Part model, mm, in its own coordinate system. A direction names the side the tool comes from. Give positions to 0.01 mm unless a question says otherwise; leave off trailing zeros. Order: outer loops, then holes, each group sorted by start corner. A loop starts at its lowest first (then second) coordinate and runs counter-clockwise, first axis right, second up. Notation, with made-up numbers: (60.5, -4.5) - (91.5, -4.5) arc R24 cw to (91.5, 26.5) - close; hole circle Ø4 at (57, 2). An arc over 180 degrees is marked (long way). One line per item, written item: value.
```python
from build123d import *

# Parameters (mm, degrees)
SKETCH1_W                       = 53.34
SKETCH1_H                       = 96.52
BOSS_EXTRUDE1_DEPTH             = 1.6002
CUT_EXTRUDE1_DEPTH              = 1.6002
F_32_0_116_DIAMETER_HOLE1_D     = 2.9464
F_32_0_116_DIAMETER_HOLE1_DEPTH = 25.4
F_32_0_116_DIAMETER_HOLE1_TIP   = 0.885187864
CUT_EXTRUDE2_DEPTH              = 2.54
FILLET1_R                       = 0.635


with BuildPart() as part:
    # Sketch1 → Boss-Extrude1 (new body)
    with BuildSketch(Plane(origin=(0, 0, 0), x_dir=(1, 0, 0), z_dir=(0, 1, 0))):
        with Locations((26.67, 48.26)):
            Rectangle(SKETCH1_W, SKETCH1_H)
    extrude(amount=BOSS_EXTRUDE1_DEPTH)

    # Sketch2 → Cut-Extrude1 (cut)
    with BuildSketch(Plane(origin=(0, 1.6002, 0), x_dir=(1, 0, 0), z_dir=(0, 1, 0))):
        Polygon((10.16, 0), (10.16, 3.81), (8.61695, 3.81), (8.61695, 6.19125), (10.16, 6.19125), (10.16, 10.16), (13.4239, 10.16), (13.4239, 6.19125), (14.96695, 6.19125), (14.96695, 3.81), (13.4239, 3.81), (13.4239, 0), align=None)
        Polygon((28.30195, 96.52), (28.30195, 92.71), (29.845, 92.71), (29.845, 90.32875), (28.30195, 90.32875), (28.30195, 86.36), (25.03805, 86.36), (25.03805, 90.32875), (23.495, 90.32875), (23.495, 92.71), (25.03805, 92.71), (25.03805, 96.52), align=None)
        Polygon((39.9161, 0), (43.18, 0), (43.18, 3.81), (44.72305, 3.81), (44.72305, 6.19125), (43.18, 6.19125), (43.18, 10.16), (39.9161, 10.16), (39.9161, 6.19125), (38.37305, 6.19125), (38.37305, 3.81), (39.9161, 3.81), align=None)
        Polygon((0, 49.911), (3.81, 49.911), (3.81, 51.435), (6.19125, 51.435), (6.19125, 49.911), (10.16, 49.911), (10.16, 46.609), (6.19125, 46.609), (6.19125, 45.085), (3.81, 45.085), (3.81, 46.609), (0, 46.609), align=None)
        Polygon((53.34, 46.609), (53.34, 49.911), (49.53, 49.911), (49.53, 51.435), (47.14875, 51.435), (47.14875, 49.911), (43.18, 49.911), (43.18, 46.609), (47.14875, 46.609), (47.14875, 45.085), (49.53, 45.085), (49.53, 46.609), align=None)
    extrude(amount=-CUT_EXTRUDE1_DEPTH, mode=Mode.SUBTRACT)

    # #32 (0.116) Diameter Hole1
    with Locations(Plane(origin=(0, 1.6002, 0), x_dir=(1, 0, 0), z_dir=(0, 1, 0))):
        with Locations((4.572, 6.35), (49.53, 22.86), (49.53, 71.12), (4.572, 67.31)):
            Hole(F_32_0_116_DIAMETER_HOLE1_D / 2, depth=F_32_0_116_DIAMETER_HOLE1_DEPTH)
            with Locations((0, 0, -(F_32_0_116_DIAMETER_HOLE1_DEPTH + F_32_0_116_DIAMETER_HOLE1_TIP / 2))):  # 118° drill point
                Cone(0, F_32_0_116_DIAMETER_HOLE1_D / 2, F_32_0_116_DIAMETER_HOLE1_TIP, mode=Mode.SUBTRACT)

    # Sketch7 → Cut-Extrude2 (cut)
    with BuildSketch(Plane(origin=(0, 1.6002, 0), x_dir=(1, 0, 0), z_dir=(0, 1, 0))):
        Polygon((26.67, 71.12), (22.426456564, 64.879494947), (24.548228282, 64.879494947), (24.548228282, 57.141268682), (26.67, 57.141268682), (28.791771718, 57.141268682), (28.791771718, 64.937563076), (30.997705847, 64.937563076), align=None)
    extrude(amount=-CUT_EXTRUDE2_DEPTH, mode=Mode.SUBTRACT)

    # Fillet1
    fillet1_edges = [part.edges().sort_by_distance(p)[0] for p in [
        (26.67, 0.8001, -71.12),
        (30.997705847, 0.8001, -64.937563076),
        (28.791771718, 0.8001, -64.937563076),
        (28.791771718, 0.8001, -57.141268682),
        (24.548228282, 0.8001, -57.141268682),
        (24.548228282, 0.8001, -64.879494947),
        (22.426456564, 0.8001, -64.879494947),
    ]]
    fillet(fillet1_edges, radius=FILLET1_R)


solid = part.part
```
1) Which spindle directions (+Z, -Z, +X, -X, +Y, -Y) get a long thin tool onto all of the face, cutting with end or side? Do faces 1 (the flat face through (24.65, 0.81, -68.15)), 2 (the flat face through (26, 1.6, -49)). Say none if no direction does.
Outcome:
face 1: +Y, -Y
face 2: +Z, -Z, +X, -X, +Y
2) Cut at D-D, the plane x = 11.5. Give the cut face in (y, z), then the cut area to 3 significant figures.
Outcome:
outline: (0, -96.52) - (1.6, -96.52) - (1.6, -10.16) - (0, -10.16) - close
area: 138 mm^2
3) Cut at A-A, the plane z = -22.86. Give the cut face in (x, y).
Outcome:
outline: (0, 0) - (48.06, 0) - (48.06, 1.6) - (0, 1.6) - close; (51, 0) - (53.34, 0) - (53.34, 1.6) - (51, 1.6) - close
4) Mould opens along X. For faces 3 (the flat face through (28.77, 0.81, -68.12)), 4 (the flat face through (26, 0, -49)) say: released by +X, released by -X, zero draft, split by the parting line, or undercut.
Outcome:
face 3: undercut
face 4: zero draft
5) Cut at B-B, the plane z = -67.31. Give the cut face in (x, y).
Outcome:
outline: (0, 0) - (3.1, 0) - (3.1, 1.6) - (0, 1.6) - close; (6.05, 0) - (24.08, 0) - (24.08, 1.6) - (6.05, 1.6) - close; (29.34, 0) - (53.34, 0) - (53.34, 1.6) - (29.34, 1.6) - close
6) Pin check, flat tip, straight feed: pin 1 (0.5 mm diameter, centred on y = 0.5, z = -2, fed in from -X). Stop position of the tip, or through.
Outcome:
pin 1: stops at x = 0
7) Cut at C-C, the plane y = 0.25. Give the number of separate pieces and of enclosed holes in the cut face, then the cut area to 3 significant figures.
Outcome:
separate pieces: 1
enclosed holes: 5
area: 4,860 mm^2
8) Drill centre lines: line 1 along X through (y, z) = (0.3, -46.5); line 2 along X through (y, z) = (0.65, -89.5); line 3 along X through (y, z) = (0.7, -6.35). Where is each one in solid material? Low to high. Write a range as from..to.
Outcome:
line 1: x = 0..3.81, 6.19..47.15, 49.53..53.34
line 2: x = 0..25.04, 28.3..53.34
line 3: x = 0..3.1, 6.05..10.16, 13.42..39.92, 43.18..53.34
